CAD build for the part. Positions are in the model's coordinates, mm. A direction names the side the tool comes from. Round coordinates to 2 decimals unless told otherwise and drop trailing zeros. Write each loop counter-clockwise with the first axis right and the second up, starting at its lowest first coordinate (ties: lowest second). Pieces come first, ordered by that corner, then holes. Notation, with made-up numbers: (41.5, -31.5) - (78.5, -31.5) arc R10 cw to (78.5, -14.5) - close; hole circle Ø2 at (-21.5, 5.25). An arc over 180 degrees is marked (long way). Put each result on its own line as item: value. Start each with the question number.
Item 1: Pin check, flat tips, straight feed: pin 1 Ø4 at (x, y) = (6.5, 15.5) entering from -Z; pin 2 Ø3 at (x, y) = (-8.5, 13) entering from -Z; pin 3 Ø8 at (y, z) = (14.5, 5) entering from -X. Stop position of each tip, or through.
Item 2: Drill centre lines: line 1 (X direction, y = 10, z = 0); line 2 (Y direction, x = 2.75, z = 10.25); line 3 (Z direction, x = 3, y = 25.5). Where is each one in solid material? Low to high. Write a range as from..to.
Item 3: Cut at A-A (y = 15). Give the cut face in (x, z), and give its area (3 significant figures).
Item 4: 3-axis set-ups, long thin cutter, end or side, ignore diameter. For faces 1 (the cylindrical face through (-10, 7, -3.2)), 2 (the cylindrical face through (-4.405, 15.902, 10.623)): which of +Z, -Z, +X, -X, +Y, -Y reach the whole face in a straight line?
Item 5: Mould opens along X. For faces 3 (the flat face through (-7, 32, 5)), 4 (the cylindrical face through (-4.405, 2.972, 10.623)), 5 (the cylindrical face through (0.33, 16.224, -7.493)) say: released by +X, released by -X, zero draft, split by the parting line, or undercut.
```python
from build123d import *

# Parameters (mm, degrees)
SKETCH1_R           = 11.5
BOSS_EXTRUDE1_DEPTH = 32
SKETCH2_R           = 7.5
CUT_EXTRUDE1_DEPTH  = 32
SKETCH3_W           = 1
SKETCH3_H           = 4
SKETCH5_W           = 1
SKETCH5_H           = 4
CHAMFER2_SIZE       = 1


with BuildPart() as part:
    # Sketch1 → Boss-Extrude1 (new body)
    with BuildSketch(Plane(origin=(0, 0, 0), x_dir=(1, 0, 0), z_dir=(0, 1, 0))):
        with Locations(Location((0, 0, 0), (0, 0, 270))):
            Circle(SKETCH1_R)
    extrude(amount=BOSS_EXTRUDE1_DEPTH)

    # Sketch2 → Cut-Extrude1 (cut)
    with BuildSketch(Plane(origin=(0, 32, 0), x_dir=(1, 0, 0), z_dir=(0, 1, 0))):
        with Locations(Location((0, 0, 0), (0, 0, 270))):
            Circle(SKETCH2_R)
    extrude(amount=-CUT_EXTRUDE1_DEPTH, mode=Mode.SUBTRACT)

    # Cut-Sweep1: sweep along a path in Sketch4
    with BuildLine(Plane(origin=(0, 7, 0), x_dir=(-1, 0, 0), z_dir=(0, -1, 0))) as cut_sweep1_path:
        CenterArc((0, 0), 11, 0, 360)
    # Sketch3 → Cut-Sweep1 (sweep, cut)
    with BuildSketch(Plane.XY):
        with Locations((11, 7)):
            Rectangle(SKETCH3_W, SKETCH3_H)
    sweep(path=cut_sweep1_path.line, mode=Mode.SUBTRACT)

    # Cut-Sweep2: sweep along a path in Sketch6
    with BuildLine(Plane(origin=(0, 25, 0), x_dir=(1, 0, 0), z_dir=(0, 1, 0))) as cut_sweep2_path:
        CenterArc((0, 0), 11, 0, 360)
    # Sketch5 → Cut-Sweep2 (sweep, cut)
    with BuildSketch(Plane(origin=(0, 0, 0), x_dir=(0, 0, -1), z_dir=(1, 0, 0))):
        with Locations((11, 25)):
            Rectangle(SKETCH5_W, SKETCH5_H)
    sweep(path=cut_sweep2_path.line, mode=Mode.SUBTRACT)

    # Chamfer2
    chamfer2_edges = [part.edges().sort_by_distance(p)[0] for p in [
        (0, 0, -11.5),
        (0, 32, -11.5),
    ]]
    chamfer(chamfer2_edges, length=CHAMFER2_SIZE)


solid = part.part
```
Output values:
1. pin 1: z = -10.58
1. pin 2: z = -9.12
1. pin 3: x = -11.46
2. line 1: -11.5..-7.5, 7.5..11.5
2. line 2: 0.11..5, 9..23, 27..31.89
2. line 3: -10.06..-6.87, 6.87..10.06
3. outline: circle Ø23 at (0, 0); hole circle Ø15 at (0, 0)
3. area: 239 mm2
4. face 1: none
4. face 2: +Y, -Y
5. face 3: zero draft
5. face 4: split by the parting line
5. face 5: undercut
